from build123d import *

# Parameters (mm, degrees)
SKETCH1_R                     = 12.7
BOSS_EXTRUDE1_DEPTH           = 31.75
FILLET1_R                     = 2.54
SKETCH3_W                     = 184.15
SKETCH3_H                     = 125
BOSS_EXTRUDE2_DEPTH           = 2.54
M5_CLEARANCE_HOLE1_AT_2_COUNT = 2
M5_CLEARANCE_HOLE1_AT_2_PITCH = 180.277563773
M5_CLEARANCE_HOLE1_AT_3_COUNT = 2
M5_CLEARANCE_HOLE1_AT_3_PITCH = 150
M5_CLEARANCE_HOLE1_AT_4_COUNT = 2
M5_CLEARANCE_HOLE1_AT_4_PITCH = 100
M5_CLEARANCE_HOLE1_AT_5_COUNT = 2
M5_CLEARANCE_HOLE1_AT_5_PITCH = 75
M5_CLEARANCE_HOLE1_AT_6_COUNT = 2
M5_CLEARANCE_HOLE1_AT_6_PITCH = 125


with BuildPart() as part:
    # Sketch1 → Boss-Extrude1 (new body)
    with BuildSketch(Plane.XY):
        Polygon((31.75, 31.75), (645.922, 31.75), (696.722, 31.75), (696.722, 0), (645.922, 0), (0, 0), (0, 336.55), (31.75, 336.55), align=None)
        with Locations((15.875, 15.875)):
            Circle(SKETCH1_R, mode=Mode.SUBTRACT)
    extrude(amount=BOSS_EXTRUDE1_DEPTH)

    # Fillet1
    fillet1_edges = [part.edges().sort_by_distance(p)[0] for p in [
        (348.361, 0, 31.75),
        (0, 168.275, 0),
        (364.236, 31.75, 31.75),
        (31.75, 184.15, 31.75),
        (0, 168.275, 31.75),
        (31.75, 184.15, 0),
        (364.236, 31.75, 0),
        (348.361, 0, 0),
    ]]
    fillet(fillet1_edges, radius=FILLET1_R)

    # Sketch3 → Boss-Extrude2 (add)
    with BuildSketch(Plane(origin=(0, 336.55, 0), x_dir=(1, 0, 0), z_dir=(0, 1, 0))):
        with Locations((92.075, -15.875)):
            Rectangle(SKETCH3_W, SKETCH3_H)
    extrude(amount=BOSS_EXTRUDE2_DEPTH)

    # Sketch8 → M5 Clearance Hole1 (revolve, cut)
    with BuildSketch(Plane(origin=(167.075, 339.09, -34.125), x_dir=(0, 0, 1), z_dir=(1, 0, 0))):
        Polygon((0, 0), (0, 2.54), (2.775, 2.54), (2.75, 2.515), (2.75, 0), align=None)
    m5_clearance_hole1 = revolve(axis=Axis((167.075, 345.44, -34.125), (0, -1, 0)), mode=Mode.SUBTRACT)

    # M5 Clearance Hole1 at 2: M5 Clearance Hole1 ×2
    with Locations(*[Vector(-0.8320502943378437, 0, 0.5547001962252293) * (i * M5_CLEARANCE_HOLE1_AT_2_PITCH) for i in range(1, M5_CLEARANCE_HOLE1_AT_2_COUNT)]):
        add(m5_clearance_hole1, mode=Mode.SUBTRACT)

    # M5 Clearance Hole1 at 3: M5 Clearance Hole1 ×2
    with Locations(*[(-i * M5_CLEARANCE_HOLE1_AT_3_PITCH, 0, 0) for i in range(1, M5_CLEARANCE_HOLE1_AT_3_COUNT)]):
        add(m5_clearance_hole1, mode=Mode.SUBTRACT)

    # M5 Clearance Hole1 at 4: M5 Clearance Hole1 ×2
    with Locations(*[(0, 0, i * M5_CLEARANCE_HOLE1_AT_4_PITCH) for i in range(1, M5_CLEARANCE_HOLE1_AT_4_COUNT)]):
        add(m5_clearance_hole1, mode=Mode.SUBTRACT)

    # M5 Clearance Hole1 at 5: M5 Clearance Hole1 ×2
    with Locations(*[(-i * M5_CLEARANCE_HOLE1_AT_5_PITCH, 0, 0) for i in range(1, M5_CLEARANCE_HOLE1_AT_5_COUNT)]):
        add(m5_clearance_hole1, mode=Mode.SUBTRACT)

    # M5 Clearance Hole1 at 6: M5 Clearance Hole1 ×2
    with Locations(*[Vector(-0.6, 0, 0.8) * (i * M5_CLEARANCE_HOLE1_AT_6_PITCH) for i in range(1, M5_CLEARANCE_HOLE1_AT_6_COUNT)]):
        add(m5_clearance_hole1, mode=Mode.SUBTRACT)


solid = part.part
The model under review builds one solid part; all positions refer to its coordinate system, in mm. A direction names the side the tool comes from. Round coordinates to 2 decimals unless told otherwise and drop trailing zeros. Order: outer loops, then holes, each group sorted by start corner. A loop starts at its lowest first (then second) coordinate and runs counter-clockwise, first axis right, second up. Notation, with made-up numbers: (41, 24) -> (70, 24) arc R25 ccw to (70, 36) -> close; hole circle Ø7 at (-22.75, 31.25). An arc over 180 degrees is marked (long way). Use CSV: the item, a comma, the result in double quotes. Start each with the question number.
(1) Mouldability with a two-part tool opening along Y and no side actions: class faces 1 (the face through (248, 22, 0)), 2 (the face through (343, 0, 16)), 3 (the face through (369, 31.75, 16)) as pulls with the +Y half, pulls with the -Y half, needs draft (parallel to the pull), parting line crosses it, or undercut.
(2) Insertion check: pin 1 (0.8 mm diameter, centred on y = 338, z = -6.5, fed in from +X); pin 2 (7 mm diameter, centred on x = 17.075, z = -34.125, fed in from +Y); pin 3 (6.5 mm diameter, centred on x = 92.075, z = 65.875, fed in from -Y); pin 4 (13.5 mm diameter, centred on x = 380, z = 12, fed in from +Y). Each pin has a flat end and moves straight along its axis. Give the tip position at first contact, or say it passes through.
(3) Tool access review of faces 4 (the face through (91, 339.09, 15)), 5 (the face through (31.75, 186, 16)), 6 (the face through (248, 22, 31.75)): name each direction out of +Z, -Z, +X, -X, +Y, -Y from which nothing blocks a thin tool from reaching the whole face with its end or side.
(4) Wall thickness on probe 1 along Y at (x, z) = (134.5, 12); probe 2 along X at (y, z) = (101, 20.5); probe 3 along Y at (x, z) = (42, -6.5): over which ranges is each line inside the solid? List them lowest first. Write a range as from..to.
(5) Consider section D-D on z = -19. Write out the cut boundary in (x, y), and give its area (3 significant figures).
(6) Consider section C-C on z = 11.5. Write out the cut boundary in (x, y) (3 decimals), and give its area (3 significant figures).
(7) Consider section A-A on y = 190.5. Write out the cut boundary in (x, z), and give its area (3 significant figures).
Responses:
1,face 1,"needs draft"
1,face 2,"pulls with the -Y half"
1,face 3,"undercut"
2,pin 1,"x = 184.15"
2,pin 2,"y = 339.09"
2,pin 3,"y = 336.55"
2,pin 4,"y = 31.75"
3,face 4,"+Z, -Z, +X, -X, +Y"
3,face 5,"+Z, -Z, +X"
3,face 6,"+Z, +X, -X, -Y"
4,probe 1,"0..31.75, 336.55..339.09"
4,probe 2,"0..31.75"
4,probe 3,"336.55..339.09"
5,outline,"(0, 336.55) -> (184.15, 336.55) -> (184.15, 339.09) -> (0, 339.09) -> close"
5,area,"468 mm²"
6,outline,"(0, 0) -> (696.722, 0) -> (696.722, 31.75) -> (31.75, 31.75) -> (31.75, 336.55) -> (184.15, 336.55) -> (184.15, 339.09) -> (0, 339.09) -> close; hole circle Ø25.4 at (15.875, 15.875)"
6,area,"31,800 mm²"
7,outline,"(0, 2.54) arc R2.54 ccw to (2.54, 0) -> (29.21, 0) arc R2.54 ccw to (31.75, 2.54) -> (31.75, 29.21) arc R2.54 ccw to (29.21, 31.75) -> (2.54, 31.75) arc R2.54 ccw to (0, 29.21) -> close"
7,area,"1,000 mm²"
